Check sheet for the drawn part. Datum: minimum x, y, z corner. Units: mm. A direction names the side the tool comes from. Give positions to 0.01 mm unless a question says otherwise; leave off trailing zeros. Write each loop counter-clockwise with the first axis right and the second up, starting at its lowest first coordinate (ties: lowest second). Pieces come first, ordered by that corner, then holes. Notation, with made-up numbers: M -32.5,-22 L 6.5,-22 A9 cw 6.5,-7 Z; hole C 86,-15.75 d11. An arc over 180 degrees is marked long. Use CSV: the item, a comma, the result in double quotes. Start each with the question number.
1. Cross-section at A-A, the plane x = 1. Enter the section's corners in (y, z).
2. Depth check by flat-ended pin: P1, Ø1.2, axis at y = 4, z = 15, coming from the -X side; P2, Ø1, axis at x = 4.5, z = 25, coming from the +Y side; P3, Ø3, axis at y = 22.5, z = 15, coming from the -X side; P4, Ø1.5, axis at x = 2, z = 5.5, coming from the +Y side (1 decimal). Enter the tip coordinate at first touch or a pass-through.
3. Scan lines: line 1 (Z direction, x = 5.5, y = 9.25) (1 decimal); line 2 (Z direction, x = 4, y = 8.5) (1 decimal); line 3 (Y direction, x = 6.75, z = 16.75) (1 decimal). Record each from-to range of solid material in increasing order.
4. Cross-section at D-D, the plane y = 21.75. Enter the section's corners in (x, z) (1 decimal).
5. Mould release check, pull along Z, two halves, no side actions. Record for the marked faces 3, 4 and 5: +Z half, -Z half, draft (parallel to the pull), parting line (faces both ways), or undercut.
6. Cross-section at B-B, the plane z = 15. Enter the section's corners in (x, y).
7. Access from +Z, -Z, +X, -X, +Y, -Y to the whole of each face (thin tool, end or side, straight path). Record for the marked faces 1 and 2.
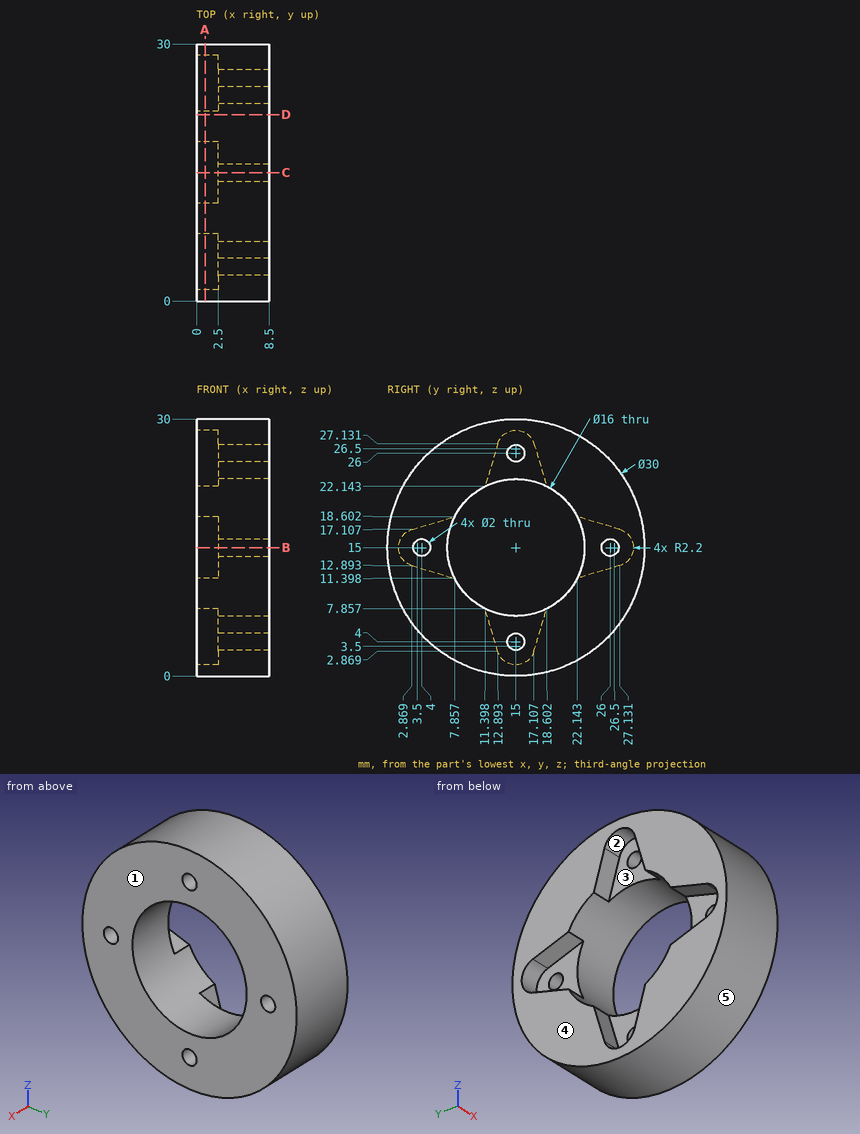
Worked answers:
1,outline,"C 15,15 d30; hole M 2.87,12.89 L 7.86,11.4 A8 ccw 11.4,7.86 L 12.89,2.87 A2.2 ccw 17.11,2.87 L 18.6,7.86 A8 ccw 22.14,11.4 L 27.13,12.89 A2.2 ccw 27.13,17.11 L 22.14,18.6 A8 ccw 18.6,22.14 L 17.11,27.13 A2.2 ccw 12.89,27.13 L 11.4,22.14 A8 ccw 7.86,18.6 L 2.87,17.11 A2.2 ccw Z"
2,P1,"passes through"
2,P2,"stops at y = 26.61"
2,P3,"stops at x = 2.5"
2,P4,"stops at y = 27.2"
3,line 1,"z = 1.1 to 9.4, 20.6 to 28.9"
3,line 2,"z = 1.5 to 10.3, 19.7 to 28.5"
3,line 3,"y = 0.1 to 7.2, 22.8 to 29.9"
4,outline,"M 0,1.6 L 8.5,1.6 L 8.5,10.7 L 0,10.7 Z; M 0,19.3 L 8.5,19.3 L 8.5,28.4 L 0,28.4 Z"
5,face 3,"undercut"
5,face 4,"draft"
5,face 5,"parting line"
6,outline,"M 0,0 L 8.5,0 L 8.5,3 L 2.5,3 L 2.5,1.3 L 0,1.3 Z; M 0,28.7 L 2.5,28.7 L 2.5,27 L 8.5,27 L 8.5,30 L 0,30 Z; M 2.5,5 L 8.5,5 L 8.5,7 L 2.5,7 Z; M 2.5,23 L 8.5,23 L 8.5,25 L 2.5,25 Z"
7,face 1,"+Z, -Z, +X, +Y, -Y"
7,face 2,"-X"
